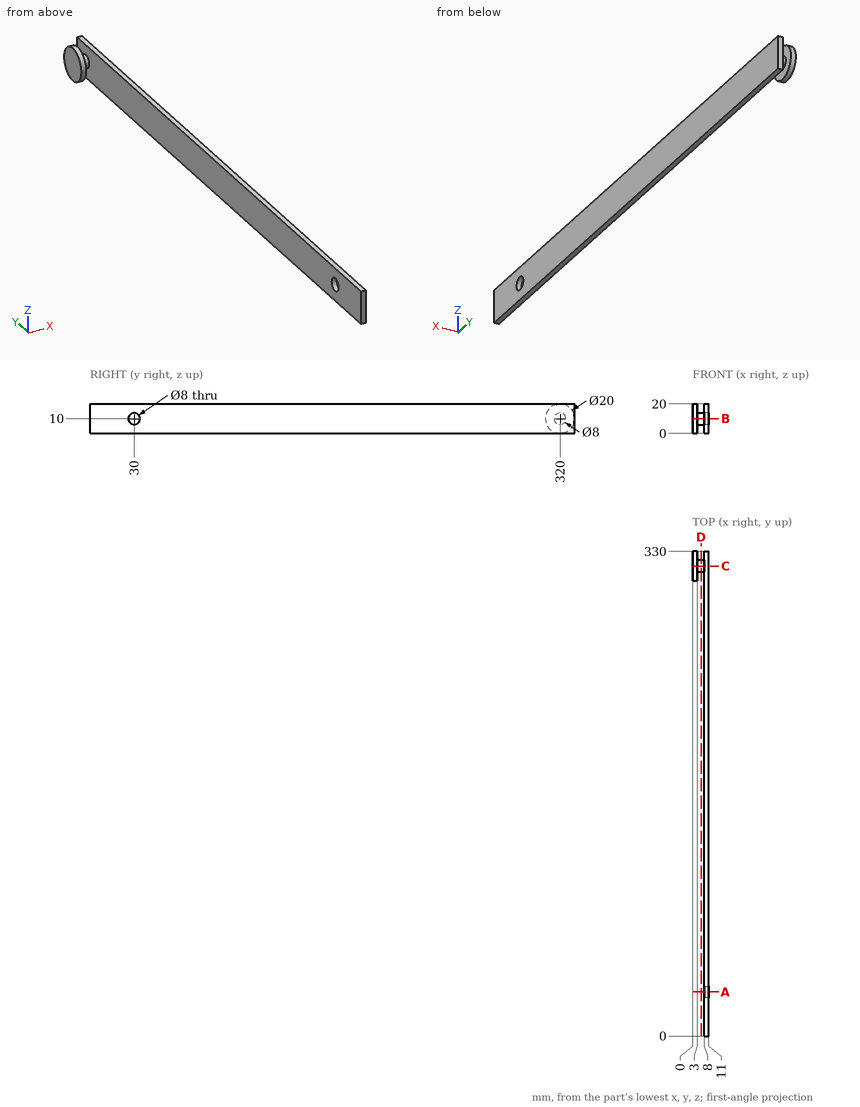
Check sheet for the drawn part. Datum: minimum x, y, z corner. Units: mm. Coordinates: 2 decimals unless noted, no trailing zeros. Loops run counter-clockwise (first coordinate to the right, second up) from the corner with the lowest first, then second, coordinate; pieces in that order, holes last. Notation, with made-up numbers: M 15,-34.75 L 67,-34.75 A21 cw 67,2.25 Z; hole C -39.75,-12 d4. An arc over 180 degrees is marked long. Answer as a JSON object with one key per item and string values.
1. Sectioned sample at C-C on y = 320. Record the cut outline in (x, z), and give its area (3 significant figures).
Outcome:
{"outline": "M 0,0 L 3,0 L 3,6 L 8,6 L 8,0 L 11,0 L 11,20 L 8,20 L 8,14 L 3,14 L 3,20 L 0,20 Z", "area": "160 mm²"}
2. Depth check by flat-ended pin: P1, Ø1.5, axis at x = 7, z = 4, coming from the -Y side; P2, Ø4, axis at x = 3.5, z = 15.5, coming from the -Y side; P3, Ø3, axis at y = 293, z = 14, coming from the -X side. Enter the tip coordinate at first touch or a pass-through.
Outcome:
{"P1": "through", "P2": "y = 310.66", "P3": "x = 8"}
3. Sectioned sample at A-A on y = 30. Record the cut outline in (x, z), and give its area (3 significant figures).
Outcome:
{"outline": "M 8,0 L 11,0 L 11,6 L 8,6 Z; M 8,14 L 11,14 L 11,20 L 8,20 Z", "area": "36.0 mm²"}
4. Sectioned sample at D-D on x = 5.75. Record the cut outline in (y, z).
Outcome:
{"outline": "C 320,10 d8"}
5. Scan lines: L1, parallel to Z at x = 9.3, y = 30; L2, parallel to X at y = 202, z = 3.5; L3, parallel to X at y = 313.5, z = 11.5. Record each from-to range of solid material in increasing order. Write a range as from..to.
Outcome:
{"L1": "0..6, 14..20", "L2": "8..11", "L3": "0..3, 8..11"}
6. Sectioned sample at B-B on z = 10. Record the cut outline in (x, y).
Outcome:
{"outline": "M 0,310 L 3,310 L 3,316 L 8,316 L 8,34 L 11,34 L 11,330 L 8,330 L 8,324 L 3,324 L 3,330 L 0,330 Z; M 8,0 L 11,0 L 11,26 L 8,26 Z"}
